```python
from build123d import *

# Parameters (mm, degrees)
BOSS_EXTRUDE1_DEPTH = 3.175
SKETCH3_R           = 2.4257
CUT_EXTRUDE2_DEPTH  = 3.175


with BuildPart() as part:
    # Sketch1 → Boss-Extrude1 (new body)
    with BuildSketch(Plane(origin=(0, 0, 0), x_dir=(1, 0, 0), z_dir=(0, 1, 0))):
        Polygon((177.8, 596.9), (63.5, 482.6), (0, 482.6), (0, 177.8), (63.5, 177.8), (177.8, 63.5), (177.8, 0), (482.6, 0), (482.6, 63.5), (596.9, 177.8), (660.4, 177.8), (660.4, 482.6), (596.9, 482.6), (482.6, 596.9), (482.6, 660.4), (177.8, 660.4), align=None)
    extrude(amount=BOSS_EXTRUDE1_DEPTH)

    # Sketch3 → Cut-Extrude2 (cut)
    with BuildSketch(Plane(origin=(0, 3.175, 0), x_dir=(1, 0, 0), z_dir=(0, 1, 0))):
        with Locations(Location((190.5, 647.7, 0), (0, 0, 270))):
            Circle(SKETCH3_R)
        with Locations(Location((260.35, 647.7, 0), (0, 0, 270))):
            Circle(SKETCH3_R)
        with Locations(Location((469.9, 647.7, 0), (0, 0, 270))):
            Circle(SKETCH3_R)
        with Locations(Location((400.05, 647.7, 0), (0, 0, 270))):
            Circle(SKETCH3_R)
        with Locations(Location((330.2, 647.7, 0), (0, 0, 270))):
            Circle(SKETCH3_R)
        with Locations(Location((647.7, 469.9, 0), (0, 0, 270))):
            Circle(SKETCH3_R)
        with Locations(Location((647.7, 400.05, 0), (0, 0, 270))):
            Circle(SKETCH3_R)
        with Locations(Location((647.7, 330.2, 0), (0, 0, 270))):
            Circle(SKETCH3_R)
        with Locations(Location((647.7, 260.35, 0), (0, 0, 270))):
            Circle(SKETCH3_R)
        with Locations(Location((647.7, 190.5, 0), (0, 0, 270))):
            Circle(SKETCH3_R)
        with Locations(Location((469.9, 12.7, 0), (0, 0, 270))):
            Circle(SKETCH3_R)
        with Locations(Location((400.05, 12.7, 0), (0, 0, 270))):
            Circle(SKETCH3_R)
        with Locations(Location((330.2, 12.7, 0), (0, 0, 270))):
            Circle(SKETCH3_R)
        with Locations(Location((260.35, 12.7, 0), (0, 0, 270))):
            Circle(SKETCH3_R)
        with Locations(Location((190.5, 12.7, 0), (0, 0, 270))):
            Circle(SKETCH3_R)
        with Locations(Location((12.7, 190.5, 0), (0, 0, 270))):
            Circle(SKETCH3_R)
        with Locations(Location((12.7, 260.35, 0), (0, 0, 270))):
            Circle(SKETCH3_R)
        with Locations(Location((12.7, 330.2, 0), (0, 0, 270))):
            Circle(SKETCH3_R)
        with Locations(Location((12.7, 400.05, 0), (0, 0, 270))):
            Circle(SKETCH3_R)
        with Locations(Location((12.7, 469.9, 0), (0, 0, 270))):
            Circle(SKETCH3_R)
    extrude(amount=-CUT_EXTRUDE2_DEPTH, mode=Mode.SUBTRACT)


solid = part.part
```
The listing builds one solid part. Answer for the finished solid, in the listing's coordinates (mm). Give positions to 0.01 mm unless a question says otherwise; leave off trailing zeros. Order: outer loops, then holes, each group sorted by start corner. A loop starts at its lowest first (then second) coordinate and runs counter-clockwise, first axis right, second up. Notation, with made-up numbers: (9.5, 89.5) -> (53.5, 89.5) arc R9 cw to (53.5, 97.5) -> close; hole circle Ø3 at (7.25, -1.5). An arc over 180 degrees is marked (long way). Answer as a JSON object with one key per item and string values. Group by question number.
Item 1: Flat-ended cylindrical pins translate along their axes: pin 1 (4 mm diameter, centred on x = 12.7, z = -190.5, fed in from -Y); pin 2 (1.6 mm diameter, centred on x = 617, y = 2, fed in from -Z); pin 3 (1 mm diameter, centred on y = 2, z = -41, fed in from +X); pin 4 (1.5 mm diameter, centred on x = 539.5, y = 1.5, fed in from -Z). Find the tip coordinate at first contact, or state that the pin passes through.
Item 2: The part is cut by section B-B on y = 2.55. Give the number of separate pieces and of enclosed holes in the cut face, and give its area (3 significant figures).
Item 3: The part is cut by section A-A on x = 538.5. Write down the section's boundary in (y, z) (3 decimals).
Item 4: Consider L1, parallel to X at y = 1.4, z = -647.7; L2, parallel to X at y = 2, z = -469.9; L3, parallel to Z at x = 260.35, y = 2.1. Determine where each line is inside the solid, lowest interval first. Write a range as from..to.
Item 5: The part is cut by section C-C on z = -578.5. Write down the section's boundary in (x, y) (3 decimals).
Result set:
{
 "1": {"pin 1": "through", "pin 2": "z = -482.6", "pin 3": "x = 482.6", "pin 4": "z = -540.75"},
 "2": {"separate pieces": "1", "enclosed holes": "20", "area": "335,000 mm²"},
 "3": {"outline": "(0, -541) -> (3.175, -541) -> (3.175, -119.4) -> (0, -119.4) -> close"},
 "4": {"L1": "177.8..188.07, 192.93..257.92, 262.78..327.77, 332.63..397.62, 402.48..467.47, 472.33..482.6", "L2": "0..10.27, 15.13..645.27, 650.13..660.4", "L3": "-660.4..-650.13, -645.27..-15.13, -10.27..0"},
 "5": {"outline": "(159.4, 0) -> (501, 0) -> (501, 3.175) -> (159.4, 3.175) -> close"}
}
